```python
from build123d import *

# Parameters (mm, degrees)
F0_R     = 25.4
F1_DEPTH = 42.42933
F2_R     = 6.35
F3_DEPTH = 12.7
F4_R     = 5.08


with BuildPart() as f1:
    # F0 (on Top) → F1 (new body)
    with BuildSketch(Plane.XY):
        Circle(F0_R)
    extrude(amount=F1_DEPTH)

    # F2 (on face) → F3 (cut)
    with BuildSketch(Plane.XY.offset(42.42933)):
        Circle(F2_R)
    extrude(amount=-F3_DEPTH, mode=Mode.SUBTRACT)

    # F4
    f4_edges = [f1.edges().sort_by_distance(p)[0] for p in [
        (-25.4, 0, 42.42933),
    ]]
    fillet(f4_edges, radius=F4_R)


solid = f1.part
```
Can you work these out from the model? Positions are in its coordinate system, mm. Round coordinates to 2 decimals unless told otherwise and drop trailing zeros. Loops run counter-clockwise (first coordinate to the right, second up) from the corner with the lowest first, then second, coordinate; pieces in that order, holes last. Notation, with made-up numbers: (76.25, 73.25) -> (83.25, 73.25) arc R21 ccw to (83.25, 97.25) -> close; hole circle Ø2 at (40, 84). An arc over 180 degrees is marked (long way). Answer in a Markdown table with one row per item.
Item 1: If I drill on probe 1 along Y at (x, z) = (0, 37.25); probe 2 along X at (y, z) = (-3, 37); probe 3 along Y at (x, z) = (0, 39.25), over which ranges is the centre line in solid material (lowest first)?
Answer block:
| item | result |
|---|---|
| probe 1 | -25.4 to -6.35, 6.35 to 25.4 |
| probe 2 | -25.22 to -5.6, 5.6 to 25.22 |
| probe 3 | -25.03 to -6.35, 6.35 to 25.03 |
Item 2: Suppose I cut it at D-D, the plane z = 36.5. List the corners of the cut face in (x, y) for me.
Answer block:
| item | result |
|---|---|
| outline | circle Ø50.8 at (0, 0); hole circle Ø12.7 at (0, 0) |
Item 3: Suppose I cut it at A-A, the plane x = 0. List the corners of the cut face in (y, z) for me.
Answer block:
| item | result |
|---|---|
| outline | (-25.4, 0) -> (25.4, 0) -> (25.4, 37.35) arc R5.08 ccw to (20.32, 42.43) -> (6.35, 42.43) -> (6.35, 29.73) -> (-6.35, 29.73) -> (-6.35, 42.43) -> (-20.32, 42.43) arc R5.08 ccw to (-25.4, 37.35) -> close |
Item 4: Suppose I cut it at C-C, the plane z = 20. List the corners of the cut face in (x, y) for me.
Answer block:
| item | result |
|---|---|
| outline | circle Ø50.8 at (0, 0) |
Item 5: We'd pull the mould along Y, two halves only. Please class faces 1 (the flat face through (0, 0, 29.729)), 2 (the cylindrical face through (-1.38, -6.2, 36.17)), 3 (the flat face through (-5, 5, 42.429)), 4 (the cylindrical face through (-5.506, -24.796, 18.413)): released by +Y, released by -Y, zero draft, split by the parting line, or undercut.
Answer block:
| item | result |
|---|---|
| face 1 | undercut |
| face 2 | undercut |
| face 3 | zero draft |
| face 4 | split by the parting line |
Item 6: Will these pins go through, and if not, where does the flat tip stop? P1, Ø2, axis at y = 17, z = 36.5, coming from the -X side; P2, Ø1.5, axis at x = -19.5, z = 16, coming from the -Y side; P3, Ø7.5, axis at x = 0, y = 0, coming from the +Z side.
Answer block:
| item | result |
|---|---|
| P1 | x = -19.73 |
| P2 | y = -17.13 |
| P3 | z = 29.73 |
